Verification items for the finished model (mm, model axes). Face numbers are marked on the shaded views. A direction names the side the tool comes from. Round coordinates to 2 decimals unless told otherwise and drop trailing zeros. Write each loop counter-clockwise with the first axis right and the second up, starting at its lowest first coordinate (ties: lowest second). Pieces come first, ordered by that corner, then holes. Notation, with made-up numbers: M 17.25,66.5 L 68.25,66.5 A31 cw 68.25,105.5 Z; hole C -16,-20 d4. An arc over 180 degrees is marked long. One line per question, with ' | ' between items.
from build123d import *

# Parameters (mm, degrees)
F1_DEPTH = 76.2
F2_R     = 5.08
F3_R     = 6.35
F4_R     = 7.14375
F5_DEPTH = 25.4


with BuildPart() as f1:
    # F0 (on Front) → F1 (new body)
    with BuildSketch(Plane.XZ):
        Polygon((-127, 0), (0, 0), (2.630256, 0), (4.490128, 1.859872), (67.351921, 64.721665), (62.861793, 69.211793), (0, 6.35), (-127, 6.35), align=None)
    extrude(amount=F1_DEPTH)

    # F2
    f2_edges = [f1.edges().sort_by_distance(p)[0] for p in [
        (0, -38.1, 6.35),
    ]]
    fillet(f2_edges, radius=F2_R)

    # F3
    f3_edges = [f1.edges().sort_by_distance(p)[0] for p in [
        (2.630256, -38.1, 0),
    ]]
    fillet(f3_edges, radius=F3_R)

    # F4 (on face) → F5 (cut)
    with BuildSketch(Plane.XY.offset(6.35)):
        with Locations((-106.3752, -38.1)):
            Circle(F4_R)
        with Locations((-68.2752, -38.1)):
            Circle(F4_R)
    extrude(amount=-F5_DEPTH, mode=Mode.SUBTRACT)


solid = f1.part
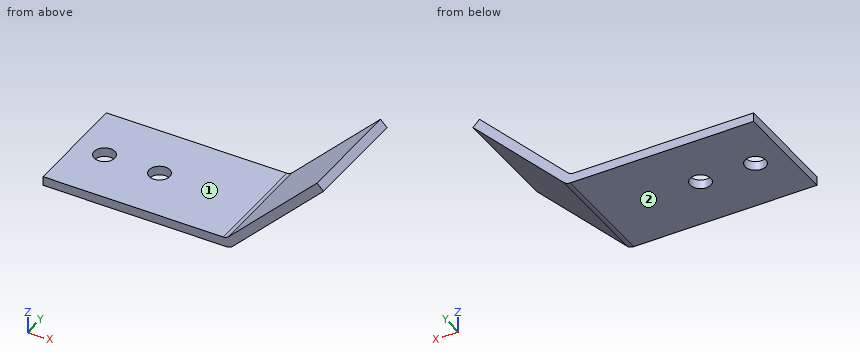
1. Section check A-A, the plane y = -38.1. Record the cut outline in (x, z).
Results:
outline: M -127,0 L -113.52,0 L -113.52,6.35 L -127,6.35 Z; M -99.23,0 L -75.42,0 L -75.42,6.35 L -99.23,6.35 Z; M -61.13,0 L 0,0 A6.35 ccw 4.49,1.86 L 67.35,64.72 L 62.86,69.21 L 1.49,7.84 A5.08 cw -2.1,6.35 L -61.13,6.35 Z
2. Go/stop test with flat-tipped pins: P1, Ø18.5, axis at x = -106.38, y = -38.1, coming from the +Z side; P2, Ø8, axis at y = -14.5, z = 38.5, coming from the -X side; P3, Ø11.5, axis at x = -68.28, y = -38.1, coming from the +Z side; P4, Ø6, axis at y = -52.5, z = 30.5, coming from the +X side. Record where each tip stops, or that it passes through.
Results:
P1: stops at z = 6.35 | P2: stops at x = 28.15 | P3: passes through | P4: stops at x = 36.13
3. Section check B-B, the plane y = -19.5. Record the cut outline in (x, z), then the cut area to 3 significant figures.
Results:
outline: M -127,0 L 0,0 A6.35 ccw 4.49,1.86 L 67.35,64.72 L 62.86,69.21 L 1.49,7.84 A5.08 cw -2.1,6.35 L -127,6.35 Z | area: 1,390 mm2
4. Thickness scan on line 1 (X direction, y = -38, z = 3); line 2 (Z direction, x = -12.5, y = -71.5); line 3 (X direction, y = -38, z = 4). Record the ranges inside material, lowest first.
Results:
line 1: x = -127 to -113.52, -99.23 to -75.42, -61.13 to 5.63 | line 2: z = 0 to 6.35 | line 3: x = -127 to -113.52, -99.23 to -75.42, -61.13 to 6.63
5. Tool access check on the marked faces 1 and 2. Record the directions out of +Z, -Z, +X, -X, +Y, -Y that give a thin tool (end or side, any length) a straight path to the whole face; none if there is none.
Results:
face 1: +Z, -X, +Y, -Y | face 2: -Z, +X, -X, +Y, -Y
6. Section check C-C, the plane x = -14.5. Record the cut outline in (y, z), then the cut area to 3 significant figures.
Results:
outline: M -76.2,0 L 0,0 L 0,6.35 L -76.2,6.35 Z | area: 484 mm2
7. Section check D-D, the plane z = 19. Record the cut outline in (x, y).
Results:
outline: M 12.65,-76.2 L 21.63,-76.2 L 21.63,0 L 12.65,0 Z
